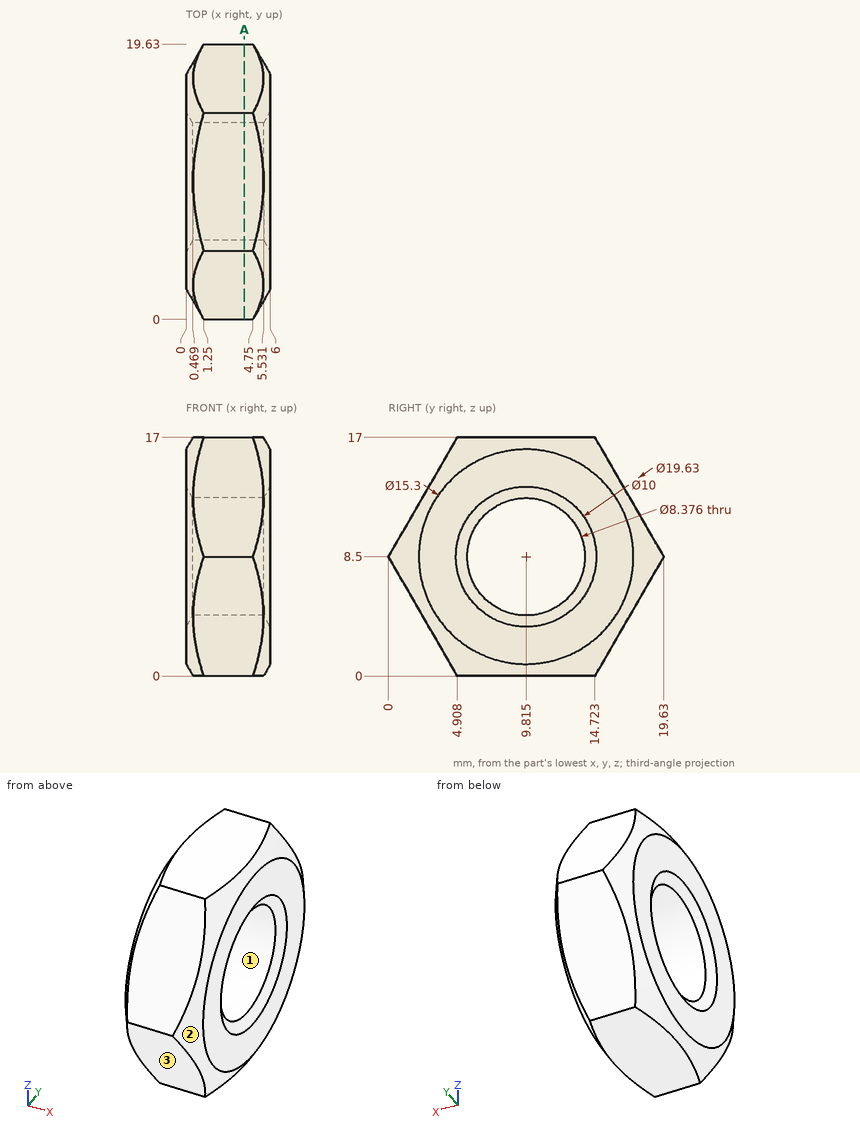
For this review, use the dimensioned drawing (mm, ordinates from the lowest corner) and the shaded views. Coordinates: 2 decimals unless noted, no trailing zeros. Loops run counter-clockwise (first coordinate to the right, second up) from the corner with the lowest first, then second, coordinate; pieces in that order, holes last.
1. For line 1 (Z direction, x = 2.65, y = 7); line 2 (Z direction, x = 0.3, y = 11.75) (1 decimal); line 3 (Y direction, x = 3.75, z = 6) (1 decimal), list the stretches that pass through material, from the lowest coordinate up.
2. Mouldability with a two-part tool opening along Y and no side actions: class the marked faces 1, 2 and 3 as +Y half, -Y half, draft (parallel to the pull), parting line (faces both ways), or undercut.
3. Add section A-A, the plane x = 4.15. Give the boundary of the cut face in (y, z) (1 decimal).
4. Insertion check: P1, Ø3, axis at x = 1, z = 12.5, coming from the -Y side; P2, Ø7.5, axis at y = 9.815, z = 8.5, coming from the +X side. Each pin has a flat end and moves straight along its axis. Give the tip position at first contact, or say it passes through.
Result:
1. line 1: z = 0 to 5.4, 11.6 to 17
1. line 2: z = 0.6 to 4.5, 12.5 to 16.4
1. line 3: y = 1.4 to 6.5, 13.2 to 18.2
2. face 1: undercut
2. face 2: parting line
2. face 3: -Y half
3. outline: (0, 8.5) - (4.9, 0) - (14.7, 0) - (19.6, 8.5) - (14.7, 17) - (4.9, 17) - close; hole circle Ø8.4 at (9.8, 8.5)
4. P1: stops at y = 1.44
4. P2: passes through
